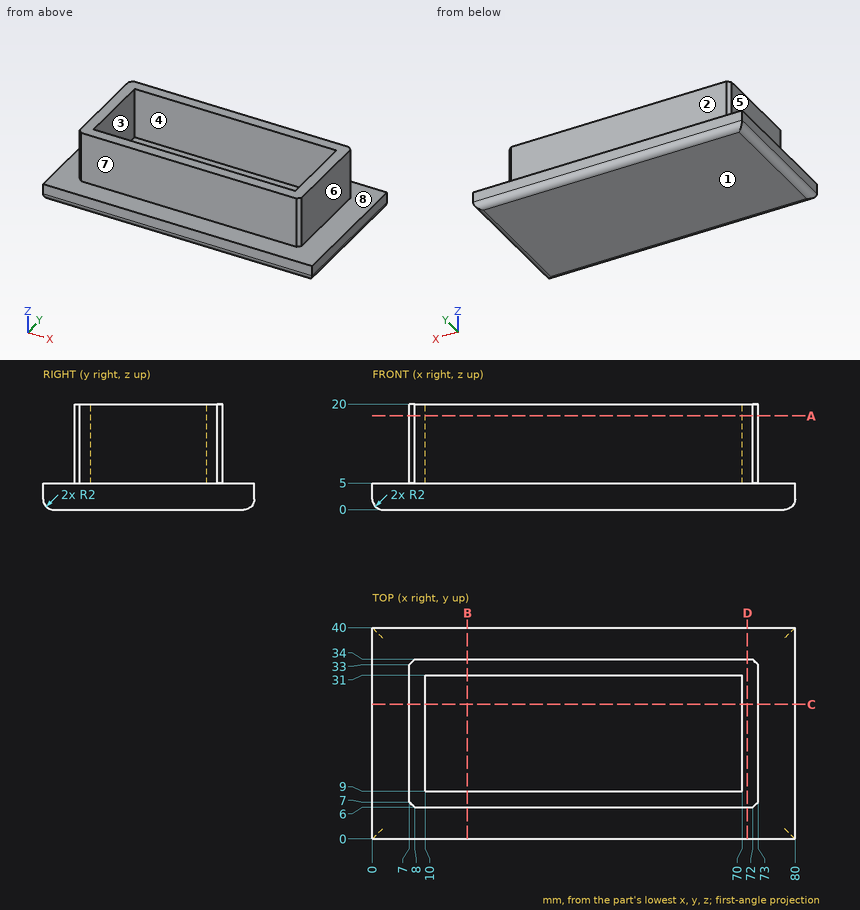
Geometry check sheet. Reference: drawing and pictorial views, mm from the part's lowest x, y, z. A direction names the side the tool comes from. Round coordinates to 2 decimals unless told otherwise and drop trailing zeros. Loops run counter-clockwise (first coordinate to the right, second up) from the corner with the lowest first, then second, coordinate; pieces in that order, holes last. Notation, with made-up numbers: (-35, 16) - (22, 16) arc R29 ccw to (22, 54) - close; hole circle Ø6 at (20.5, -2). An arc over 180 degrees is marked (long way). Use a Markdown table: item, result.
Q1. Go/stop test with flat-tipped pins: P1, Ø4.5, axis at x = 24.5, z = 13, coming from the -Y side; P2, Ø17.5, axis at x = 33, y = 20, coming from the +Z side; P3, Ø4, axis at y = 16, z = 15, coming from the -X side. Record where each tip stops, or that it passes through.
Solutions:
| item | result |
|---|---|
| P1 | stops at y = 6 |
| P2 | stops at z = 5 |
| P3 | stops at x = 7 |
Q2. Cross-section at D-D on x = 71. Record the cut outline in (y, z), plus the area to 3 significant figures.
Solutions:
| item | result |
|---|---|
| outline | (0, 2) arc R2 ccw to (2, 0) - (38, 0) arc R2 ccw to (40, 2) - (40, 5) - (34, 5) - (34, 20) - (6, 20) - (6, 5) - (0, 5) - close |
| area | 618 mm2 |
Q3. Cross-section at A-A on z = 17.75. Record the cut outline in (x, y).
Solutions:
| item | result |
|---|---|
| outline | (7, 7) - (8, 6) - (72, 6) - (73, 7) - (73, 33) - (72, 34) - (8, 34) - (7, 33) - close; hole (10, 9) - (70, 9) - (70, 31) - (10, 31) - close |
Q4. Material ranges on line 1 (Y direction, x = 64, z = 12.75); line 2 (X direction, y = 17.5, z = 16); line 3 (Z direction, x = 10.5, y = 12), recorded low to high.
Solutions:
| item | result |
|---|---|
| line 1 | y = 6 to 9, 31 to 34 |
| line 2 | x = 7 to 10, 70 to 73 |
| line 3 | z = 0 to 5 |
Q5. Cross-section at B-B on x = 18. Record the cut outline in (y, z).
Solutions:
| item | result |
|---|---|
| outline | (0, 2) arc R2 ccw to (2, 0) - (38, 0) arc R2 ccw to (40, 2) - (40, 5) - (34, 5) - (34, 20) - (31, 20) - (31, 5) - (9, 5) - (9, 20) - (6, 20) - (6, 5) - (0, 5) - close |
Q6. Draft check along Y on the marked faces 1, 2, 3 and 4. Enter one of: released by +Y, released by -Y, zero draft, split by the parting line, or undercut.
Solutions:
| item | result |
|---|---|
| face 1 | zero draft |
| face 2 | released by +Y |
| face 3 | undercut |
| face 4 | undercut |
Q7. Cross-section at C-C on y = 25.5. Record the cut outline in (x, z), plus the area to 3 significant figures.
Solutions:
| item | result |
|---|---|
| outline | (0, 2) arc R2 ccw to (2, 0) - (78, 0) arc R2 ccw to (80, 2) - (80, 5) - (73, 5) - (73, 20) - (70, 20) - (70, 5) - (10, 5) - (10, 20) - (7, 20) - (7, 5) - (0, 5) - close |
| area | 488 mm2 |
Q8. Access from +Z, -Z, +X, -X, +Y, -Y to the whole of each face (thin tool, end or side, straight path). Record for the marked faces 5, 6, 7 and 8.
Solutions:
| item | result |
|---|---|
| face 5 | +Z, -X, +Y, -Y |
| face 6 | +Z, +X, +Y, -Y |
| face 7 | +Z, +X, -X, -Y |
| face 8 | +Z |
